Study the drawing (mm; zero at the part's minimum x, y, z) and answer. Round coordinates to 2 decimals unless told otherwise and drop trailing zeros. Write each loop counter-clockwise with the first axis right and the second up, starting at its lowest first coordinate (ties: lowest second). Pieces come first, ordered by that corner, then holes. Notation, with made-up numbers: (79.25, -37) - (120.25, -37) arc R28 cw to (120.25, -7) - close; hole circle Ø9 at (-27, -0.5). An arc over 180 degrees is marked (long way). Use one line per item in the form item = value. Start each with the question number.
1) The part is cut by section A-A, the plane y = 14. Give the vertices of the cut face in (x, z), plus the area to 3 significant figures.
2) Consider line 1 along X through (y, z) = (46, 43); line 2 along Y through (x, z) = (16, 20). Determine where each line is inside the solid, lowest interval first. Write a range as from..to.
3) The part is cut by section C-C, the plane z = 28. Give the vertices of the cut face in (x, y).
4) The part is cut by section B-B, the plane x = 53. Give the vertices of the cut face in (y, z).
5) For a pull along Z with two mould halves and no side action, classify the marked faces 1, 2, 3 and 4 as released by +Z, released by -Z, zero draft, split by the parting line, or undercut.
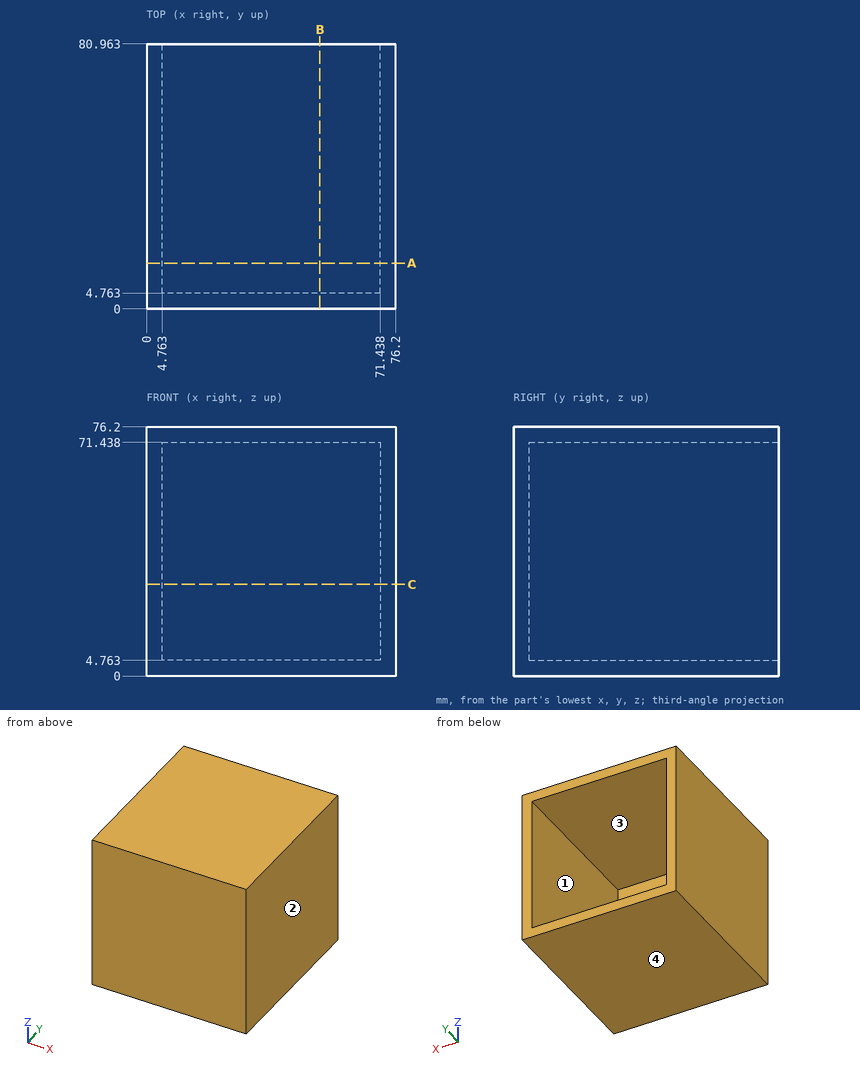
Geometry results:
q1.outline = (0, 0) - (76.2, 0) - (76.2, 76.2) - (0, 76.2) - close; hole (4.76, 4.76) - (71.44, 4.76) - (71.44, 71.44) - (4.76, 71.44) - close
q1.area = 1,360 mm2
q2.line_1 = 0..4.76, 71.44..76.2
q2.line_2 = 0..4.76
q3.outline = (0, 0) - (76.2, 0) - (76.2, 80.96) - (71.44, 80.96) - (71.44, 4.76) - (4.76, 4.76) - (4.76, 80.96) - (0, 80.96) - close
q4.outline = (0, 0) - (80.96, 0) - (80.96, 4.76) - (4.76, 4.76) - (4.76, 71.44) - (80.96, 71.44) - (80.96, 76.2) - (0, 76.2) - close
q5.face_1 = undercut
q5.face_2 = zero draft
q5.face_3 = undercut
q5.face_4 = released by -Z
